Could you check a few things on this model? Use its own coordinates, in mm. A direction names the side the tool comes from. Round coordinates to 2 decimals unless told otherwise and drop trailing zeros. Loops run counter-clockwise (first coordinate to the right, second up) from the corner with the lowest first, then second, coordinate; pieces in that order, holes last. Notation, with made-up numbers: (23, -3) - (44, -3) arc R9 ccw to (44, 11) - close; hole circle Ø11 at (-17.75, 83.25). An arc over 180 degrees is marked (long way). Answer as CSV lines item,"result". Start each with the question number.
1) I'm going to push flat-ended pins straight in: pin 1 Ø10 at (x, z) = (-7, 29) entering from -Y; pin 2 Ø22.5 at (x, y) = (-17, 34.5) entering from +Z; pin 3 Ø24 at (x, z) = (-20.5, 38.5) entering from +Y. Where does each tip first touch, or does it pass through?
2) Suppose I cut it at D-D, the plane x = -33. Write out the boundary of the cut face in (y, z), then the cut area to 3 significant figures.
3) Which directions (+Z, -Z, +X, -X, +Y, -Y) give clear straight access to the entire face, cutting with the end or side of a thin tool? Please do faces 5 (the face through (-47, 49, 1)), 6 (the face through (-39.9, 1.41, 10.75)), 7 (the face through (-47.2, 9, 6)).
4) Please list where these lines run through material, in increasing order: line 1 along Y through (x, z) = (-40.5, 1.55); line 2 along Y through (x, z) = (-9.5, 1); line 3 along X through (y, z) = (15, 1).
5) We'd pull the mould along X, two halves only. Please class faces 1 (the face through (0, 11, 10)), 2 (the face through (-25, 2.85, 30)), 3 (the face through (-47, 1, 52)), 4 (the face through (-10.1, 1.4, 45)): pulls with the +X half, pulls with the -X half, needs draft (parallel to the pull), parting line crosses it, or undercut.
6) Suppose I cut it at C-C, the plane x = -39.85. Write out the boundary of the cut face in (y, z), then the cut area to 3 significant figures.
7) Suppose I cut it at B-B, the plane y = 31. Write out the boundary of the cut face in (x, z), then the cut area to 3 significant figures.
8) Suppose I cut it at A-A, the plane z = 38.5. Write out the boundary of the cut face in (x, y).
Autodesk Inventor part; units mm, degrees
ref_plane "YZ Plane" through (0, 0, 0) normal (1, 0, 0) x (0, 1, 0)
ref_plane "XZ Plane" through (0, 0, 0) normal (0, 1, 0) x (-1, 0, 0)
ref_plane "XY Plane" through (0, 0, 0) normal (0, 0, 1) x (1, 0, 0)
sketch "Sketch1" plane through (0, 0, 0) normal (1, 0, 0) x (0, 1, 0)
  line L0 (3, 0) -> (51, 0)
  line L1 (51, 0) -> (51, 2.85)
  line L2 (51, 2.85) -> (5.85, 2.85)
  line L3 (2.85, 5.85) -> (2.85, 54)
  line L4 (2.85, 54) -> (0, 54)
  line L5 (0, 54) -> (0, 3)
  arc A0 (0, 3) -> (3, 0) centre (3, 3) ccw
  arc A1 (2.85, 5.85) -> (5.85, 2.85) centre (5.85, 5.85) ccw
  point P0 (0, 0)
  dimension "d0" = 51
  dimension "d1" = 2.85
  dimension "d2" = 2.85
  dimension "d3" = 54
  dimension "d4" = 3
extrude "Extrusion1" add sketch "Sketch1" against normal blind 50
sketch "Sketch2" plane through (0, 0, 0) normal (1, 0, 0) x (0, 0, -1)
  line L0 (-54, 2.85) -> (-54, 0)
  line L1 (-54, 0) -> (-3, 0)
  arc A0 (-3, 0) -> (0, 3) centre (-3, 3) ccw
  line L2 (0, 3) -> (0, 51)
  line L3 (0, 51) -> (-2.85, 51)
  line L4 (-2.85, 51) -> (-2.85, 5.85)
  arc A1 (-5.85, 2.85) -> (-2.85, 5.85) centre (-5.85, 5.85) ccw
  line L5 (-5.85, 2.85) -> (-54, 2.85)
  line L6 (-5.85, 2.85) -> (-54, 2.85)
  line L7 (-15.85, 2.85) -> (-2.85, 22.85)
  line L8 (-2.85, 51) -> (-2.85, 5.85)
  point P0 (0, 0)
  point P1 (-2.85, 22.85)
  dimension "d7" = 20
  dimension "d8" = 13
extrude "Extrusion2" add sketch "Sketch2" against normal blind 2.8 contours L7 L4 A1 L5
sketch "Sketch3" plane through (-50, 0, 0) normal (-1, 0, 0) x (0, 0, 1)
  line L0 (2.85, 5.85) -> (2.85, 22.85)
  arc A0 (2.85, 5.85) -> (5.85, 2.85) centre (5.85, 5.85) ccw
  line L1 (15.85, 2.85) -> (5.85, 2.85)
  line L2 (15.85, 2.85) -> (2.85, 22.85)
  point P0 (0, 0)
extrude "Extrusion3" add sketch "Sketch3" against normal blind 2.8
sketch "Sketch4" plane through (0, 3, 0) normal (0, 0, -1) x (-1, 0, 0)
  line L0 (0, 48) -> (50, 48) construction
  line L1 (25, 48) -> (25, -3) construction
  line L2 (0, -3) -> (50, -3) construction
  line L3 (0, 48) -> (0, 19.85) construction
  line L4 (0, 28) -> (50, 28) construction
  line L5 (50, 48) -> (50, 0) construction
  circle A0 centre (25, 28) radius 11
  line L6 (9.5, 43.5) -> (40.5, 43.5) construction
  line L7 (40.5, 43.5) -> (40.5, 12.5) construction
  line L8 (40.5, 12.5) -> (9.5, 12.5) construction
  line L9 (9.5, 12.5) -> (9.5, 43.5) construction
  circle A1 centre (9.5, 43.5) radius 1.8
  circle A2 centre (40.5, 43.5) radius 1.8
  circle A3 centre (40.5, 12.5) radius 1.8
  circle A4 centre (9.5, 12.5) radius 1.8
  dimension "d13" = 20
  dimension "d14" = 22
  dimension "d15" = 31
  dimension "d16" = 31
  dimension "d17" = 3.6
  dimension "d18" = 3.6
  dimension "d19" = 3.6
  dimension "d20" = 3.6
  dimension "d21" = 15.5
  dimension "d22" = 15.5
extrude "Extrusion4" cut sketch "Sketch4" against normal up to next
sketch "Sketch5" plane through (0, 0, 3) normal (0, -1, 0) x (1, 0, 0)
  line L0 (0, 51) -> (-50, 51) construction
  line L1 (-38.7, -3) -> (-42.3, -3) construction
  line L2 (-39.85, 51) -> (-39.85, -3.09) construction
  line L3 (0, -3) -> (-50, -3) construction
  line L4 (-50, 0) -> (-50, 51) construction
  line L5 (-25, 51) -> (-25, -3) construction
  line L6 (-39.85, 42) -> (-39.85, 7.75) construction
  line L7 (-42, 39.85) -> (-42, 9.9)
  line L8 (-37.7, 9.9) -> (-37.7, 39.85)
  arc A0 (-37.7, 39.85) -> (-42, 39.85) centre (-39.85, 39.85) ccw
  arc A1 (-42, 9.9) -> (-37.7, 9.9) centre (-39.85, 9.9) ccw
  line L9 (-10.15, 42) -> (-10.15, 7.75) construction
  line L10 (-8, 39.85) -> (-8, 9.9)
  line L11 (-12.3, 9.9) -> (-12.3, 39.85)
  arc A2 (-8, 39.85) -> (-12.3, 39.85) centre (-10.15, 39.85) ccw
  arc A3 (-12.3, 9.9) -> (-8, 9.9) centre (-10.15, 9.9) ccw
  point P0 (-39.85, 24.875)
  point P1 (-10.15, 24.875)
  dimension "d25" = 10.15
  dimension "d26" = 34.25
  dimension "d27" = 4.3
  dimension "d28" = 9
extrude "Extrusion5" cut sketch "Sketch5" against normal up to next
chamfer "Chamfer1" distance 5 angle 45 4 edges at (0, 1.425, 54) (-50, 1.425, 54) (-50, 51, 1.425) (0, 51, 1.425)
equation "\"d2\" = d1"
equation "\"d18\" = d17"
equation "\"d19\" = d17"
equation "\"d20\" = d17"
equation "\"d21\" = 0.5 * d15"
equation "\"d22\" = 0.5 * d16"
properties part number "Nema 17 Stepper Motor Mounting Bracket"
Filled sheet:
1,pin 1,"y = 0"
1,pin 2,"z = 2.85"
1,pin 3,"y = 2.85"
2,outline,"(0, 3) arc R3 ccw to (3, 0) - (23.45, 0) - (23.45, 2.85) - (5.85, 2.85) arc R3 cw to (2.85, 5.85) - (2.85, 54) - (0, 54) - close; (38.55, 0) - (51, 0) - (51, 2.85) - (38.55, 2.85) - close"
2,area,"248 mm²"
3,face 5,"+Z, -Z, -X, +Y"
3,face 6,"+Y, -Y"
3,face 7,"+Z, +Y"
4,line 1,"0.37 to 13.7, 17.3 to 44.7, 48.3 to 51"
4,line 2,"0.76 to 13.7, 17.3 to 44.7, 48.3 to 51"
4,line 3,"-50 to -42.23, -38.77 to -11.23, -7.77 to 0"
5,face 1,"pulls with the +X half"
5,face 2,"undercut"
5,face 3,"pulls with the -X half"
5,face 4,"undercut"
6,outline,"(0, 3) arc R3 ccw to (3, 0) - (13.82, 0) - (13.82, 2.85) - (5.85, 2.85) arc R3 cw to (2.85, 5.85) - (2.85, 10.75) - (0, 10.75) - close; (0, 45) - (2.85, 45) - (2.85, 54) - (0, 54) - close; (17.18, 0) - (44.82, 0) - (44.82, 2.85) - (17.18, 2.85) - close; (48.18, 0) - (51, 0) - (51, 2.85) - (48.18, 2.85) - close"
6,area,"174 mm²"
7,outline,"(-50, 0) - (-36, 0) - (-36, 2.85) - (-50, 2.85) - close; (-14, 0) - (0, 0) - (0, 2.85) - (-14, 2.85) - close"
7,area,"79.8 mm²"
8,outline,"(-50, 0) - (-42, 0) - (-42, 2.85) - (-50, 2.85) - close; (-37.7, 0) - (-12.3, 0) - (-12.3, 2.85) - (-37.7, 2.85) - close; (-8, 0) - (0, 0) - (0, 2.85) - (-8, 2.85) - close"
